```python
from build123d import *

# Parameters (mm, degrees)
F0_W          = 20.846172
F0_H          = 3.5
F0_W_2        = 3
F0_H_2        = 6.2
F1_DEPTH      = 3.9
F1_DEPTH_BACK = 3.9
F2_R          = 1.75
F3_DEPTH      = 16.2
F5_DEPTH      = 8
F5_DEPTH_BACK = 8
F6_R          = 7
F7_R          = 1.5
F8_DEPTH      = 25
F9_R          = 1.5
F10_DEPTH     = 1


with BuildPart() as f1:
    # F0 (on Top) → F1 (new body, two sides)
    with BuildSketch(Plane.XY) as f1_sk:
        with BuildLine():
            Line((-17.5, 8), (-17.5, -8))
            Line((-17.5, -8), (13.5, -8))
            ThreePointArc((13.5, -8), (16.328427, -6.828427), (17.5, -4))
            Line((17.5, -4), (17.5, 4))
            ThreePointArc((17.5, 4), (16.328427, 6.828427), (13.5, 8))
            Line((13.5, 8), (-17.5, 8))
        make_face()
        with Locations((-3.937322, 0)):
            Rectangle(F0_W, F0_H, mode=Mode.SUBTRACT)
        with Locations((12, 0)):
            Rectangle(F0_W_2, F0_H_2, mode=Mode.SUBTRACT)
    extrude(amount=F1_DEPTH)
    extrude(f1_sk.sketch, amount=-F1_DEPTH_BACK)

    # F2 (on face) → F3 (cut)
    with BuildSketch(Plane.YZ.offset(17.5)):
        Circle(F2_R)
    extrude(amount=-F3_DEPTH, mode=Mode.SUBTRACT)

    # F4 (on Front) → F5 (join, two sides)
    with BuildSketch(Plane.XZ) as f5_sk:
        with BuildLine():
            Line((-22.917766, 3.95), (-22.917766, -3.95))
            ThreePointArc((-22.917766, -3.95), (-23.210659, -4.657107), (-23.917766, -4.95))
            Line((-23.917766, -4.95), (-37.917766, -4.95))
            Line((-37.917766, -4.95), (-37.917766, -8.95))
            Line((-37.917766, -8.95), (-20.07043, -8.95))
            Line((-20.07043, -8.95), (-16.954886, -3.836561))
            Line((-16.954886, -3.836561), (-16.954886, 3.836561))
            Line((-16.954886, 3.836561), (-20.07043, 8.95))
            Line((-20.07043, 8.95), (-37.917766, 8.95))
            Line((-37.917766, 8.95), (-37.917766, 4.95))
            Line((-37.917766, 4.95), (-23.917766, 4.95))
            ThreePointArc((-23.917766, 4.95), (-23.210659, 4.657107), (-22.917766, 3.95))
        make_face()
    extrude(amount=F5_DEPTH)
    extrude(f5_sk.sketch, amount=-F5_DEPTH_BACK)

    # F6
    f6_edges = [f1.edges().sort_by_distance(p)[0] for p in [
        (-37.917766, -8, -6.95),
        (-37.917766, -8, 6.95),
        (-37.917766, 8, 6.95),
        (-37.917766, 8, -6.95),
    ]]
    fillet(f6_edges, radius=F6_R)

    # F7 (on face) → F8 (cut)
    with BuildSketch(Plane(origin=(0, 0, -8.95), x_dir=(1, 0, 0), z_dir=(0, 0, -1))):
        with Locations((-30.917766, 0)):
            Circle(F7_R)
    extrude(amount=-F8_DEPTH, mode=Mode.SUBTRACT)

    # F9 (on face) → F10 (cut)
    with BuildSketch(Plane(origin=(0, 0, -8.95), x_dir=(1, 0, 0), z_dir=(0, 0, -1))):
        Polygon((-29.417766, -2.598076), (-27.917766, 0), (-29.417766, 2.598076), (-32.417766, 2.598076), (-33.917766, 0), (-32.417766, -2.598076), align=None)
        with Locations((-30.917766, 0)):
            Circle(F9_R, mode=Mode.SUBTRACT)
    extrude(amount=-F10_DEPTH, mode=Mode.SUBTRACT)


solid = f1.part
```
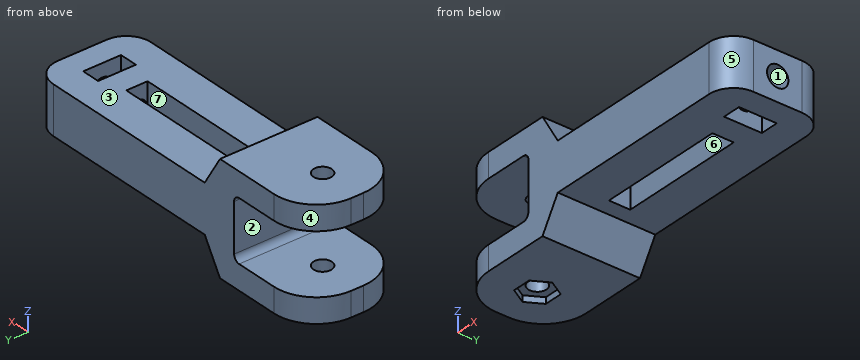
Geometry check sheet. Reference: the model listing, model coordinates, mm. Face numbers are marked on the shaded views. A direction names the side the tool comes from. Give positions to 0.01 mm unless a question says otherwise; leave off trailing zeros. Order: outer loops, then holes, each group sorted by start corner. A loop starts at its lowest first (then second) coordinate and runs counter-clockwise, first axis right, second up. Notation, with made-up numbers: (-5, -39.75) -> (8, -39.75) arc R17 ccw to (8, -33.75) -> close; hole circle Ø4 at (-39.5, 74). An arc over 180 degrees is marked (long way). Write each question's results on one line, items separated by ' | '. Start each with the question number.
(1) Sectioned sample at D-D (y = -5.75). Enter the section's corners in (x, z), plus the area to 3 significant figures.
(2) Sectioned sample at B-B (z = 2.75). Enter the section's corners in (x, y), plus the area to 3 significant figures.
(3) Scan lines: line 1 (Y direction, x = 7.75, z = 0); line 2 (Z direction, x = -35, y = -1.5). Record each from-to range of solid material in increasing order.
(4) Access from +Z, -Z, +X, -X, +Y, -Y to the whole of each face (thin tool, end or side, straight path). Record for the marked faces 1, 2 and 3.
(5) Sectioned sample at A-A (x = 12.5). Enter the section's corners in (y, z).
(6) Mould release check, pull along X, two halves, no side actions. Record for the marked faces 4, 5, 6 and 7: pulls with the +X half, pulls with the -X half, needs draft (parallel to the pull), parting line crosses it, or undercut.
(7) Gauge pin test, flat ends, axial feed: P1, Ø1, axis at y = 0.5, z = -1.5, coming from the -X side; P2, Ø4.5, axis at y = 0, z = 0, coming from the +X side; P3, Ø1, axis at y = 0, z = 1, coming from the +X side; P4, Ø3, axis at x = -11.5, y = 2, coming from the +Z side. Record the tip position at first contact, or that the pin passes through.
(8) Sectioned sample at C-C (x = 2.5). Enter the section's corners in (y, z), plus the area to 3 significant figures.
Answer below:
1) outline: (-36.06, -8.95) -> (-20.07, -8.95) -> (-16.99, -3.9) -> (17.1, -3.9) -> (17.1, 3.9) -> (-16.99, 3.9) -> (-20.07, 8.95) -> (-36.06, 8.95) -> (-36.06, 4.95) -> (-23.92, 4.95) arc R1 cw to (-22.92, 3.95) -> (-22.92, -3.95) arc R1 cw to (-23.92, -4.95) -> (-36.06, -4.95) -> close | area: 462 mm2
2) outline: (-22.92, -8) -> (13.5, -8) arc R4 ccw to (17.5, -4) -> (17.5, 4) arc R4 ccw to (13.5, 8) -> (-22.92, 8) -> close; hole (-14.36, -1.75) -> (6.49, -1.75) -> (6.49, 1.75) -> (-14.36, 1.75) -> close; hole (10.5, -3.1) -> (13.5, -3.1) -> (13.5, 3.1) -> (10.5, 3.1) -> close | area: 548 mm2
3) line 1: -8 to -1.75, 1.75 to 8 | line 2: -8.95 to -4.95, 4.95 to 8.95
4) face 1: +X | face 2: -X, +Y, -Y | face 3: +Z, +X, +Y, -Y
5) outline: (-8, -3.9) -> (-3.1, -3.9) -> (-3.1, 3.9) -> (-8, 3.9) -> close; (3.1, -3.9) -> (8, -3.9) -> (8, 3.9) -> (3.1, 3.9) -> close
6) face 4: pulls with the -X half | face 5: pulls with the +X half | face 6: undercut | face 7: undercut
7) P1: x = -22.92 | P2: x = 17.5 | P3: x = -14.36 | P4: z = 3.9
8) outline: (-8, -3.9) -> (-1.75, -3.9) -> (-1.75, 3.9) -> (-8, 3.9) -> close; (1.75, -3.9) -> (8, -3.9) -> (8, 3.9) -> (1.75, 3.9) -> close | area: 97.5 mm2
